Verification items for this drawing (mm, ordinates from the low corner). Round coordinates to 2 decimals unless told otherwise and drop trailing zeros. Loops run counter-clockwise (first coordinate to the right, second up) from the corner with the lowest first, then second, coordinate; pieces in that order, holes last. Notation, with made-up numbers: (-5, 31.5) -> (38, 31.5) arc R18 ccw to (38, 35.5) -> close; hole circle Ø5 at (35, -27). An arc over 180 degrees is marked (long way). Use a Markdown table: item, result. Add a question column.
Q1. Sectioned sample at B-B, the plane y = 8.25. Enter the section's corners in (x, z), then the cut area to 3 significant figures.
Q2. Material ranges on L1, parallel to Z at x = 87, y = 9.75; L2, parallel to Z at x = 55, y = 6; L3, parallel to Z at x = 31.5, y = 10.5, recorded low to high.
Q3. Sectioned sample at A-A, the plane x = 70. Enter the section's corners in (y, z), then the cut area to 3 significant figures.
Q4. Sectioned sample at C-C, the plane x = 23.5. Enter the section's corners in (y, z).
Q5. Gauge pin test, flat ends, axial feed: P1, Ø4, axis at x = 52.5, y = 9, coming from the -Z side; P2, Ø1, axis at y = 11, z = 70, coming from the +X side. Record the tip position at first contact, or that the pin passes through.
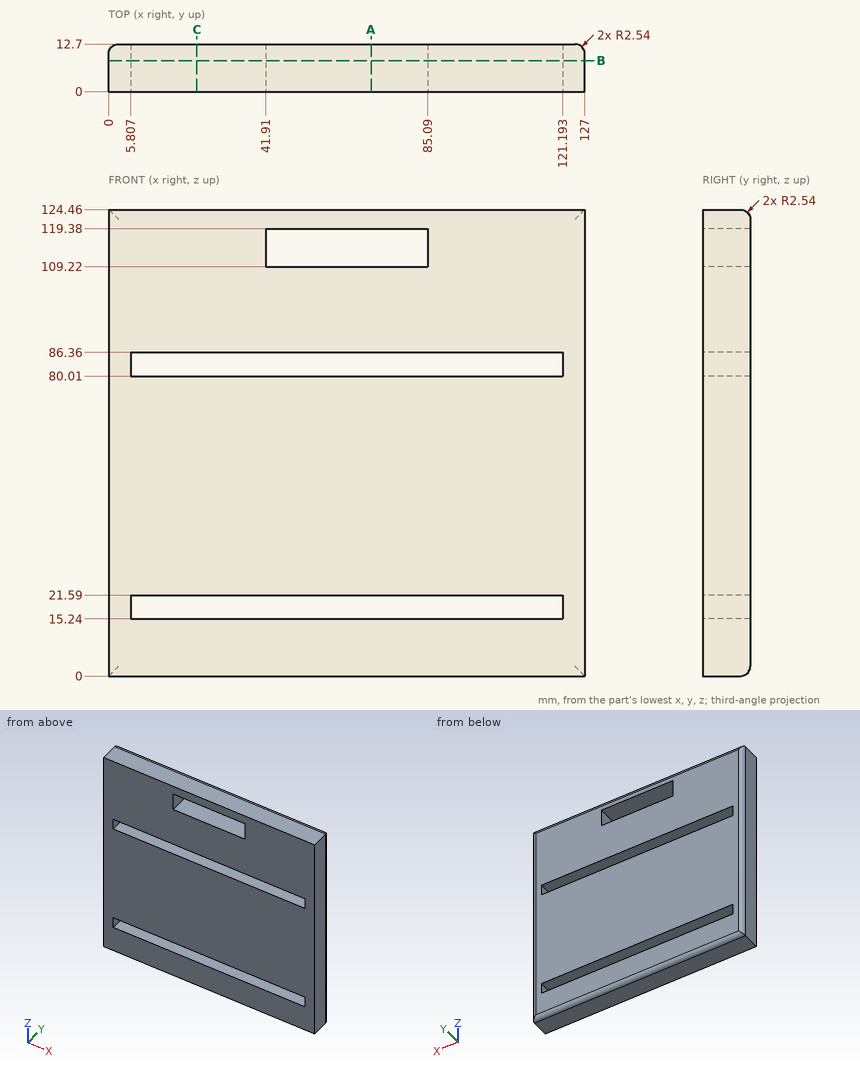
Values:
| question | item | result |
|---|---|---|
| 1 | outline | (0, 0) -> (127, 0) -> (127, 124.46) -> (0, 124.46) -> close; hole (5.81, 15.24) -> (121.19, 15.24) -> (121.19, 21.59) -> (5.81, 21.59) -> close; hole (5.81, 80.01) -> (121.19, 80.01) -> (121.19, 86.36) -> (5.81, 86.36) -> close; hole (41.91, 109.22) -> (85.09, 109.22) -> (85.09, 119.38) -> (41.91, 119.38) -> close |
| 1 | area | 13,900 mm^2 |
| 2 | L1 | 0 to 15.24, 21.59 to 80.01, 86.36 to 124.46 |
| 2 | L2 | 0 to 15.24, 21.59 to 80.01, 86.36 to 109.22, 119.38 to 124.46 |
| 2 | L3 | 0.02 to 15.24, 21.59 to 80.01, 86.36 to 124.44 |
| 3 | outline | (0, 0) -> (10.16, 0) arc R2.54 ccw to (12.7, 2.54) -> (12.7, 15.24) -> (0, 15.24) -> close; (0, 21.59) -> (12.7, 21.59) -> (12.7, 80.01) -> (0, 80.01) -> close; (0, 86.36) -> (12.7, 86.36) -> (12.7, 109.22) -> (0, 109.22) -> close; (0, 119.38) -> (12.7, 119.38) -> (12.7, 121.92) arc R2.54 ccw to (10.16, 124.46) -> (0, 124.46) -> close |
| 3 | area | 1,290 mm^2 |
| 4 | outline | (0, 0) -> (10.16, 0) arc R2.54 ccw to (12.7, 2.54) -> (12.7, 15.24) -> (0, 15.24) -> close; (0, 21.59) -> (12.7, 21.59) -> (12.7, 80.01) -> (0, 80.01) -> close; (0, 86.36) -> (12.7, 86.36) -> (12.7, 121.92) arc R2.54 ccw to (10.16, 124.46) -> (0, 124.46) -> close |
| 5 | P1 | z = 0 |
| 5 | P2 | x = 126.98 |
